```python
from build123d import *

# Parameters (mm, degrees)
SKETCH1_R           = 1.6
SKETCH1_R_2         = 0.9
BOSS_EXTRUDE1_DEPTH = 3.5
CUT_EXTRUDE1_DEPTH  = 2.3


with BuildPart() as part:
    # Sketch1 → Boss-Extrude1 (new body)
    with BuildSketch(Plane(origin=(0, 0, 0), x_dir=(1, 0, 0), z_dir=(0, 1, 0))):
        with BuildLine():
            Line((0, 0), (61.25, 0))
            Line((61.25, 0), (61.25, 4))
            ThreePointArc((61.25, 4), (65, 7.75), (68.75, 4))
            Line((68.75, 4), (68.75, 0))
            Line((68.75, 0), (130, 0))
            Line((130, 0), (130, -100))
            Line((130, -100), (111.5, -100))
            Line((111.5, -100), (111.5, -110))
            Line((111.5, -110), (116.5, -110))
            Line((116.5, -110), (116.5, -160))
            Line((116.5, -160), (111.5, -160))
            Line((111.5, -160), (111.5, -115))
            Line((111.5, -115), (106.5, -115))
            Line((106.5, -115), (106.5, -110))
            Line((106.5, -110), (106.5, -100))
            Line((106.5, -100), (76.5, -100))
            Line((76.5, -100), (76.5, -110))
            Line((76.5, -110), (76.5, -115))
            Line((76.5, -115), (71.5, -115))
            Line((71.5, -115), (71.5, -160))
            Line((71.5, -160), (66.5, -160))
            Line((66.5, -160), (66.5, -110))
            Line((66.5, -110), (71.5, -110))
            Line((71.5, -110), (71.5, -100))
            Line((71.5, -100), (68.75, -100))
            Line((68.75, -100), (68.75, -104))
            ThreePointArc((68.75, -104), (65, -107.75), (61.25, -104))
            Line((61.25, -104), (61.25, -100))
            Line((61.25, -100), (0, -100))
            Line((0, -100), (0, 0))
        make_face()
        with Locations(Location((65, 4, 0), (0, 0, 270))):
            Circle(SKETCH1_R, mode=Mode.SUBTRACT)
        with Locations(Location((65, -104, 0), (0, 0, 270))):
            Circle(SKETCH1_R, mode=Mode.SUBTRACT)
        with Locations(Location((114.5, -112, 0), (0, 0, 270))):
            Circle(SKETCH1_R_2, mode=Mode.SUBTRACT)
        with Locations(Location((114.5, -158, 0), (0, 0, 270))):
            Circle(SKETCH1_R_2, mode=Mode.SUBTRACT)
        with Locations(Location((68.5, -158, 0), (0, 0, 270))):
            Circle(SKETCH1_R_2, mode=Mode.SUBTRACT)
        with Locations(Location((68.5, -112, 0), (0, 0, 270))):
            Circle(SKETCH1_R_2, mode=Mode.SUBTRACT)
    extrude(amount=BOSS_EXTRUDE1_DEPTH)

    # Sketch2 → Cut-Extrude1 (cut)
    with BuildSketch(Plane(origin=(0, 3.5, 0), x_dir=(1, 0, 0), z_dir=(0, 1, 0))):
        Polygon((3.212435565, -2), (2.606217783, -0.95), (1.393782217, -0.95), (0.787564435, -2), (1.393782217, -3.05), (2.606217783, -3.05), align=None)
        Polygon((126.787564435, -2), (127.393782217, -3.05), (128.606217783, -3.05), (129.212435565, -2), (128.606217783, -0.95), (127.393782217, -0.95), align=None)
        Polygon((126.787564435, -98), (127.393782217, -99.05), (128.606217783, -99.05), (129.212435565, -98), (128.606217783, -96.95), (127.393782217, -96.95), align=None)
        Polygon((3.212435565, -98), (2.606217783, -96.95), (1.393782217, -96.95), (0.787564435, -98), (1.393782217, -99.05), (2.606217783, -99.05), align=None)
    extrude(amount=-CUT_EXTRUDE1_DEPTH, mode=Mode.SUBTRACT)


solid = part.part
```
Part model, mm, in its own coordinate system. A direction names the side the tool comes from. Give positions to 0.01 mm unless a question says otherwise; leave off trailing zeros. Write each loop counter-clockwise with the first axis right and the second up, starting at its lowest first coordinate (ties: lowest second). Pieces come first, ordered by that corner, then holes. Notation, with made-up numbers: (81, 71.25) -> (88, 71.25) arc R25 cw to (88, 108.25) -> close; hole circle Ø11 at (28, 79). An arc over 180 degrees is marked (long way). Put each result on its own line as item: value. Start each with the question number.
Item 1: Which spindle directions (+Z, -Z, +X, -X, +Y, -Y) get a long thin tool onto all of the face, cutting with end or side? Do faces 1 (the face through (76.5, 2, 107)), 2 (the face through (61.25, 2, -2)), 3 (the face through (114, 2, 110)), 4 (the face through (69, 2, 110)). Say none if no direction does.
Item 2: Cut at A-A (z = 144). List the corners of the cut face in (x, y), then the cut area to 3 significant figures.
Item 3: Pull direction X, two halves, no side cores. Call faces 5 (the face through (68.75, 2, -2)), 6 (the face through (111.5, 2, 138)), 7 (the face through (0, 2, 51)), 8 (the face through (65.08, 1.73, 107.75)): pulls with the +X half, pulls with the -X half, needs draft (parallel to the pull), parting line crosses it, or undercut.
Item 4: Cut at D-D (x = 74.5). List the corners of the cut face in (y, z).
Item 5: Cut at B-B (y = 1.75). State how many separate pieces and enclosed holes the cut face has, then the cut area to 3 significant figures.
Item 6: Wall check: L1, parallel to X at y = 1.4, z = 101; L2, parallel to X at y = 1.8, z = 158; L3, parallel to X at y = 2.1, z = 144.5. Give the ranges that are in metal, low to high. Write a range as [from, to].
Item 7: Pin check, flat tips, straight feed: pin 1 Ø0.6 at (x, z) = (128.5, 2) entering from +Y; pin 2 Ø1.5 at (x, z) = (106.5, 115.5) entering from +Y; pin 3 Ø0.6 at (x, y) = (127.5, 2.5) entering from -Z; pin 4 Ø1 at (y, z) = (1, -2) entering from -X. Stop position of each tip, or through.
Item 8: Cut at C-C (x = 119.5). List the corners of the cut face in (y, z).
Answer list:
1. face 1: +Z, +Y, -Y
1. face 2: -Z, -X, +Y, -Y
1. face 3: +X, +Y, -Y
1. face 4: -X, +Y, -Y
2. outline: (66.5, 0) -> (71.5, 0) -> (71.5, 3.5) -> (66.5, 3.5) -> close; (111.5, 0) -> (116.5, 0) -> (116.5, 3.5) -> (111.5, 3.5) -> close
2. area: 35.0 mm2
3. face 5: pulls with the +X half
3. face 6: undercut
3. face 7: pulls with the -X half
3. face 8: undercut
4. outline: (0, 0) -> (3.5, 0) -> (3.5, 115) -> (0, 115) -> close
5. separate pieces: 1
5. enclosed holes: 10
5. area: 13,700 mm2
6. L1: x = [61.25, 68.75], [71.5, 76.5], [106.5, 111.5]
6. L2: x = [66.5, 67.6], [69.4, 71.5], [111.5, 113.6], [115.4, 116.5]
6. L3: x = [66.5, 71.5], [111.5, 116.5]
7. pin 1: stops at y = 1.2
7. pin 2: stops at y = 3.5
7. pin 3: stops at z = 0
7. pin 4: stops at x = 61.25
8. outline: (0, 0) -> (3.5, 0) -> (3.5, 100) -> (0, 100) -> close
